Can you work these out from the drawing? Everything is in mm from the part's minimum corner. A direction names the side the tool comes from. Coordinates: 2 decimals unless noted, no trailing zeros. Order: outer loops, then holes, each group sorted by start corner. A loop starts at its lowest first (then second) coordinate and runs counter-clockwise, first axis right, second up. Notation, with made-up numbers: (76.25, 54.5) - (127.25, 54.5) arc R12 cw to (127.25, 75.5) - close; hole circle Ø5 at (-34, 83.5). An arc over 180 degrees is marked (long way). Answer as CSV lines item,"result". Start each with the question number.
Item 1: On a 3-axis mill with a long thin cutter (end or side, diameter ignored), from which of +Z, -Z, +X, -X, +Y, -Y can I reach the whole of each face in a straight line? I mean the marked faces 1, 2 and 3. Say none if no direction works.
Item 2: Imagine slicing it at A-A on z = 80. List the corners of the cut face in (x, y) for me, and give its area (4 significant figures).
Item 3: Imagine slicing it at D-D on y = 254.5. List the corners of the cut face in (x, z) for me.
Item 4: I'm going to push flat-ended pins straight in: pin 1 (10 mm diameter, centred on x = 22, y = 251, fed in from -Z); pin 2 (6 mm diameter, centred on y = 238.5, z = 61, fed in from +X); pin 3 (10 mm diameter, centred on x = 45.5, z = 79.5, fed in from -Y); pin 4 (1 mm diameter, centred on x = 46.5, y = 248, fed in from +Z). Where does each tip first touch, or does it pass through?
Item 5: Imagine slicing it at C-C on x = 52.5. List the corners of the cut face in (y, z) for me, and give its area (3 significant figures).
Item 6: I need wall thicknesses on line 1 (Z direction, x = 121, y = 145.5); line 2 (X direction, y = 181, z = 127); line 3 (Y direction, x = 50, z = 32.5). Which ranges of each line are inside material? Lowest first, please.
Item 7: Imagine slicing it at B-B on y = 57.5. List the corners of the cut face in (x, z) for me.
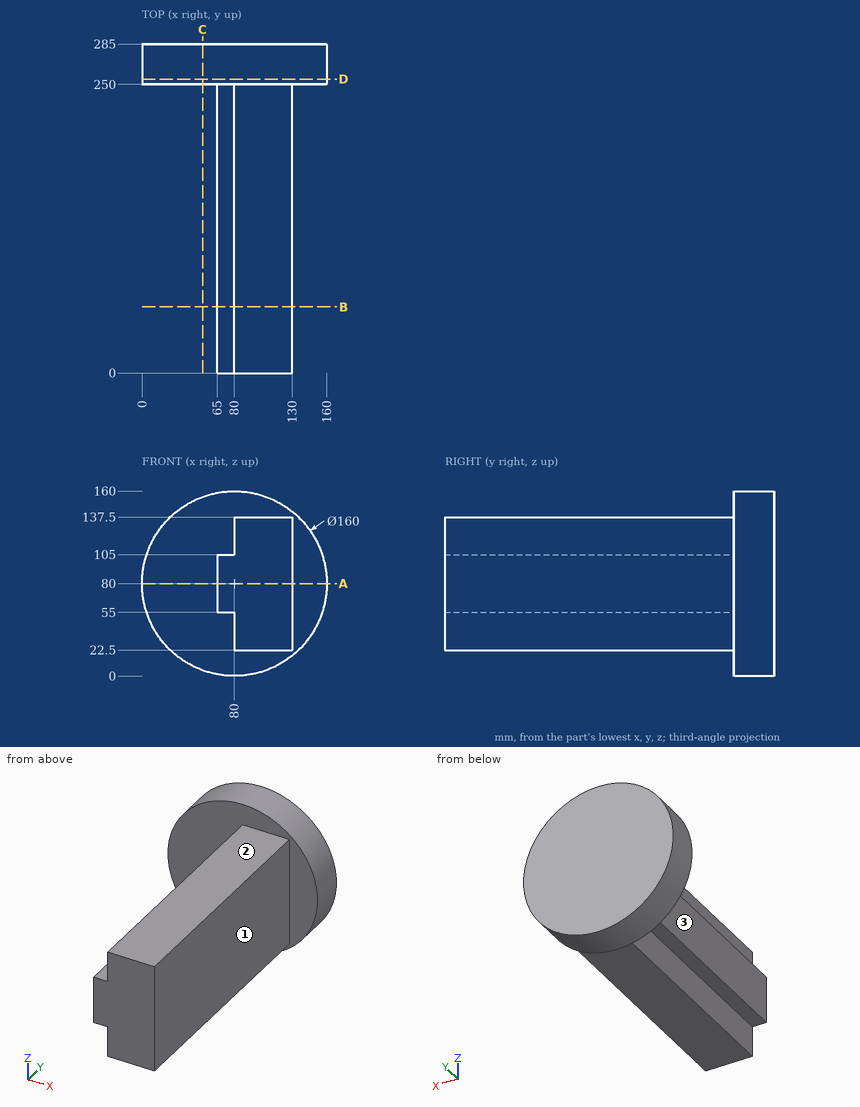
Responses:
1,face 1,"+Z, -Z, +X, -Y"
1,face 2,"+Z, +X, -X, -Y"
1,face 3,"+Z, -Z, -X, -Y"
2,outline,"(0, 250) - (65, 250) - (65, 0) - (130, 0) - (130, 250) - (160, 250) - (160, 285) - (0, 285) - close"
2,area,"21,850 mm^2"
3,outline,"circle Ø160 at (80, 80)"
4,pin 1,"stops at z = 20.08"
4,pin 2,"stops at x = 130"
4,pin 3,"stops at y = 250"
4,pin 4,"passes through"
5,outline,"(250, 4.88) - (285, 4.88) - (285, 155.12) - (250, 155.12) - close"
5,area,"5,260 mm^2"
6,line 1,"z = 22.5 to 137.5"
6,line 2,"x = 80 to 130"
6,line 3,"y = 250 to 285"
7,outline,"(65, 55) - (80, 55) - (80, 22.5) - (130, 22.5) - (130, 137.5) - (80, 137.5) - (80, 105) - (65, 105) - close"
